Can you work these out from the model? Positions are in its coordinate system, mm. A direction names the side the tool comes from. Give positions to 0.01 mm unless a question says otherwise; leave off trailing zeros. Write each loop counter-clockwise with the first axis right and the second up, starting at its lowest first coordinate (ties: lowest second). Pieces come first, ordered by that corner, then holes. Notation, with made-up numbers: (27.5, 78.25) -> (80.5, 78.25) arc R22 cw to (80.5, 91.25) -> close; hole circle Ø1 at (59.25, -9). An arc over 180 degrees is marked (long way). Answer as CSV lines item,"result". Start each with the question number.
1. If we section it at C-C on z = 50: Write out the boundary of the cut face in (x, y) (3 decimals), plus the area to 3 significant figures.
2. If we section it at D-D on x = 66: Write out the boundary of the cut face in (y, z) (3 decimals).
3. On a 3-axis mill with a long thin cutter (end or side, diameter ignored), from which of +Z, -Z, +X, -X, +Y, -Y can I reach the whole of each face in a straight line? I mean faces 4 (the face through (-10.96, 2.58, -16.6)), 5 (the face through (-0.071, 1.565, -10.732)), 6 (the face through (-1.069, 7.656, 66.666)). Say none if no direction works.
4. If we mould it in two halves opening along Z, with no side actions, what happens to faces 1 (the face through (2, 10.16, 0)), 2 (the face through (-48.077, 5.142, -0.216)), 3 (the face through (-46.367, 6.619, -60.47))? For each: pulls with the +Z half, pulls with the -Z half, needs draft (parallel to the pull), parting line crosses it, or undercut.
5. If we section it at B-B on x = -43.18: Write out the boundary of the cut face in (y, z) (3 decimals).
6. If we section it at A-A on x = 0: Write out the boundary of the cut face in (y, z) (1 decimal).
7. I'm going to push flat-ended pins straight in: P1, Ø3, axis at x = 55, y = 8.5, coming from the -Z side; P2, Ø1.9, axis at x = 1, z = 23.5, coming from the -Y side (3 decimals); P3, Ø3.5, axis at x = 24.49, z = 29.19, coming from the +Y side; P4, Ø1.6, axis at x = -29.19, z = 24.49, coming from the +Y side. Where does each tip first touch, or does it pass through?
8. I need wall thicknesses on line 1 (X direction, y = 7.75, z = 0); line 2 (Z direction, x = -10, y = 5.25); line 3 (Z direction, x = 56.5, y = 5.25). Which ranges of each line are inside material? Lowest first, please. Write a range as [from, to].
```python
from build123d import *

# Parameters (mm, degrees)
SKETCH1_R                      = 76.2
BOSS_EXTRUDE1_DEPTH            = 10.16
TAP_DRILL_FOR_6_32_TAP1_D      = 2.7051
CIRPATTERN1_COUNT              = 4
W_0_386_DIAMETER_HOLE1_D       = 9.8044
F_3_16_0_1875_DIAMETER_HOLE1_D = 4.7625
CUT_EXTRUDE4_DEPTH             = 3.175
SKETCH15_R                     = 76.2
SKETCH15_R_2                   = 74.041
CUT_EXTRUDE5_DEPTH             = 3.175
CUT_EXTRUDE7_DEPTH             = 5.08
BODY_MOVE_COPY1_ANGLE          = 40
CHAMFER1_SIZE                  = 0.635


with BuildPart() as part:
    # Sketch1 → Boss-Extrude1 (new body)
    with BuildSketch(Plane(origin=(0, 0, 0), x_dir=(1, 0, 0), z_dir=(0, 1, 0))):
        with Locations(Location((0, 0, 0), (0, 0, 270))):
            Circle(SKETCH1_R)
    extrude(amount=BOSS_EXTRUDE1_DEPTH)

    # Tap Drill for #6-32 Tap1 (through all)
    with Locations(Plane(origin=(0, 0, 0), x_dir=(-1, 0, 0), z_dir=(0, -1, 0))):
        with Locations((37.52117539, 6.615995569)):
            tap_drill_for_6_32_tap1 = Hole(TAP_DRILL_FOR_6_32_TAP1_D / 2)

    # CirPattern1: Tap Drill for #6-32 Tap1 ×4 about axis, 1 skipped
    cirpattern1_axis = Axis((0, 0, 0), (0, 1, 0))
    add([tap_drill_for_6_32_tap1.rotate(cirpattern1_axis, i * 360 / CIRPATTERN1_COUNT) for i in range(1, CIRPATTERN1_COUNT) if i not in (3,)], mode=Mode.SUBTRACT)

    # W (0.386) Diameter Hole1 (through all)
    with Locations(Plane(origin=(0, 0, 0), x_dir=(-1, 0, 0), z_dir=(0, -1, 0))):
        with Locations((-33.077799054, 27.755568986), (33.077799054, -27.755568986)):
            Hole(W_0_386_DIAMETER_HOLE1_D / 2)

    # 3/16 (0.1875) Diameter Hole1 (through all)
    with Locations(Plane(origin=(0, 0, 0), x_dir=(-1, 0, 0), z_dir=(0, -1, 0))):
        with Locations((18.760587695, 3.307997785)):
            Hole(F_3_16_0_1875_DIAMETER_HOLE1_D / 2)

    # Sketch12 → Cut-Extrude4 (cut)
    with BuildSketch(Plane.XZ):
        with BuildLine():
            ThreePointArc((24.848558171, 24.575146858), (20.286055568, 24.175979603), (19.886888313, 28.738482206))
            Line((19.886888313, 28.738482206), (6.498907978, 12.783308544))
            ThreePointArc((6.498907978, 12.783308544), (10.087375141, 13.744835423), (12.218242907, 10.70164087))
            ThreePointArc((12.218242907, 10.70164087), (12.02293746, 9.594008636), (11.460577836, 8.619973196))
            Line((11.460577836, 8.619973196), (24.848558171, 24.575146858))
        make_face()
        with BuildLine():
            ThreePointArc((25.606223242, 26.656814532), (23.475355476, 29.700009084), (19.886888313, 28.738482206))
            Line((19.886888313, 28.738482206), (24.848558171, 24.575146858))
            ThreePointArc((24.848558171, 24.575146858), (25.410917794, 25.549182297), (25.606223242, 26.656814532))
        make_face()
        with BuildLine():
            Line((24.848558171, 24.575146858), (19.886888313, 28.738482206))
            ThreePointArc((19.886888313, 28.738482206), (20.286055568, 24.175979603), (24.848558171, 24.575146858))
        make_face()
        with BuildLine():
            ThreePointArc((12.218242907, 10.70164087), (10.087375141, 13.744835423), (6.498907978, 12.783308544))
            Line((6.498907978, 12.783308544), (11.460577836, 8.619973196))
            ThreePointArc((11.460577836, 8.619973196), (12.02293746, 9.594008636), (12.218242907, 10.70164087))
        make_face()
        with BuildLine():
            Line((11.460577836, 8.619973196), (6.498907978, 12.783308544))
            ThreePointArc((6.498907978, 12.783308544), (6.898075233, 8.220805941), (11.460577836, 8.619973196))
        make_face()
    cut_extrude4 = extrude(amount=-CUT_EXTRUDE4_DEPTH, mode=Mode.SUBTRACT)

    # Mirror1: Cut-Extrude4 across plane
    add(cut_extrude4.mirror(Plane(origin=(0, 0, 0), x_dir=(-0.7660444431189792, 0, 0.6427876096865378), z_dir=(0.6427876096865379, 0, 0.7660444431189792))), mode=Mode.SUBTRACT)

    # Sketch15 → Cut-Extrude5 (cut)
    with BuildSketch(Plane.XZ):
        with Locations(Location((0, 0, 0), (0, 0, 270))):
            Circle(SKETCH15_R)
        with Locations(Location((0, 0, 0), (0, 0, 270))):
            Circle(SKETCH15_R_2, mode=Mode.SUBTRACT)
    extrude(amount=-CUT_EXTRUDE5_DEPTH, mode=Mode.SUBTRACT)

    # Sketch20 → Cut-Extrude7 (cut)
    with BuildSketch(Plane(origin=(0, 10.16, 0), x_dir=(1, 0, 0), z_dir=(0, 1, 0))):
        with BuildLine():
            Line((58.006337644, 21.112580301), (15.787325383, 5.746116518))
            ThreePointArc((15.787325383, 5.746116518), (13.41810781, 3.858627578), (12.666324636, 0.92424034))
            ThreePointArc((12.666324636, 0.92424034), (8.163402625, -9.728764443), (-3.109683289, -12.313402042))
            ThreePointArc((-3.109683289, -12.313402042), (-6.130036388, -12.544212982), (-8.400260426, -14.549677855))
            Line((-8.400260426, -14.549677855), (-30.864527746, -53.458930208))
            ThreePointArc((-30.864527746, -53.458930208), (-31.28945063, -57.248955123), (-28.797011077, -60.135578304))
            ThreePointArc((-28.797011077, -60.135578304), (42.857863777, -51.076013328), (64.222532311, 17.917085938))
            ThreePointArc((64.222532311, 17.917085938), (61.812570917, 20.872916849), (58.006337644, 21.112580301))
        make_face()
        with BuildLine():
            Line((8.400260408, 14.549677823), (30.864527463, 53.458929718))
            ThreePointArc((30.864527463, 53.458929718), (31.289450636, 57.248955104), (28.797010604, 60.135578531))
            ThreePointArc((28.797010604, 60.135578531), (-42.857863971, 51.076013165), (-64.222532316, -17.91708592))
            ThreePointArc((-64.222532316, -17.91708592), (-61.812570882, -20.872916867), (-58.006337553, -21.112580268))
            Line((-58.006337553, -21.112580268), (-15.787325417, -5.746116531))
            ThreePointArc((-15.787325417, -5.746116531), (-13.418107797, -3.858627558), (-12.666324642, -0.924240256))
            ThreePointArc((-12.666324642, -0.924240256), (-8.16340261, 9.728764456), (3.109683246, 12.313402053))
            ThreePointArc((3.109683246, 12.313402053), (6.130036351, 12.544212967), (8.400260408, 14.549677823))
        make_face()
    extrude(amount=-CUT_EXTRUDE7_DEPTH, mode=Mode.SUBTRACT)


with BuildPart() as part_1:
    # Body-Move/Copy1: moved
    add(part.part.rotate(Axis((0, 0, 0), (0, -1, 0)), BODY_MOVE_COPY1_ANGLE))

    # Chamfer1
    chamfer1_edges = [part_1.edges().sort_by_distance(p)[0] for p in [
        (-46.935303069, 0, -3.15107342),
        (-46.935303069, 10.16, -3.15107342),
        (39.424696931, 0, -3.15107342),
        (39.424696931, 10.16, -3.15107342),
    ]]
    chamfer(chamfer1_edges, length=CHAMFER1_SIZE)


solid = part_1.part
```
Computed values:
1,outline,"(-57.502, 3.175) -> (-54.608, 3.175) -> (-54.608, 0) -> (54.608, 0) -> (54.608, 3.175) -> (57.502, 3.175) -> (57.502, 10.16) -> (44.108, 10.16) -> (44.108, 5.08) -> (-44.108, 5.08) -> (-44.108, 10.16) -> (-57.502, 10.16) -> close"
1,area,"702 mm2"
2,outline,"(0, -33.557) -> (3.175, -33.557) -> (3.175, -38.085) -> (10.16, -38.085) -> (10.16, 38.085) -> (3.175, 38.085) -> (3.175, 33.557) -> (0, 33.557) -> close"
3,face 4,"+Y, -Y"
3,face 5,"-Y"
3,face 6,"+Y"
4,face 1,"needs draft"
4,face 2,"undercut"
4,face 3,"parting line crosses it"
5,outline,"(0, -60.146) -> (3.175, -60.146) -> (3.175, -62.785) -> (10.16, -62.785) -> (10.16, -50.804) -> (5.08, -50.804) -> (5.08, -15.716) -> (10.16, -15.716) -> (10.16, -5.537) -> (9.525, -4.902) -> (0.635, -4.902) -> (0, -5.537) -> close; (0, 5.537) -> (0.635, 4.902) -> (9.525, 4.902) -> (10.16, 5.537) -> (10.16, 15.716) -> (5.08, 15.716) -> (5.08, 50.804) -> (10.16, 50.804) -> (10.16, 62.785) -> (3.175, 62.785) -> (3.175, 60.146) -> (0, 60.146) -> close"
6,outline,"(0, -74) -> (3.2, -74) -> (3.2, -76.2) -> (10.2, -76.2) -> (10.2, -66.7) -> (5.1, -66.7) -> (5.1, -12.7) -> (10.2, -12.7) -> (10.2, 12.7) -> (5.1, 12.7) -> (5.1, 66.7) -> (10.2, 66.7) -> (10.2, 76.2) -> (3.2, 76.2) -> (3.2, 74) -> (0, 74) -> (0, 38) -> (3.2, 38) -> (3.2, 10.7) -> (0, 10.7) -> (0, -10.7) -> (3.2, -10.7) -> (3.2, -38) -> (0, -38) -> close"
7,P1,"stops at z = -54.26"
7,P2,"stops at y = 3.175"
7,P3,"stops at y = 5.08"
7,P4,"passes through"
8,line 1,"x = [-76.2, -48.08], [-38.28, 38.28], [48.08, 76.2]"
8,line 2,"z = [-75.54, -65.92], [-7.83, 7.83], [65.92, 75.54]"
8,line 3,"z = [-51.13, -35.4], [-20.56, 20.56], [35.4, 51.13]"
